Design review of the part built by this model. Coordinates are the model's own, in mm. A direction names the side the tool comes from. Give positions to 0.01 mm unless a question says otherwise; leave off trailing zeros. Write each loop counter-clockwise with the first axis right and the second up, starting at its lowest first coordinate (ties: lowest second). Pieces come first, ordered by that corner, then holes. Notation, with made-up numbers: (16.25, 63) -> (51.25, 63) arc R27 cw to (51.25, 95) -> close; hole circle Ø11 at (13, -32.75). An arc over 180 degrees is marked (long way). Return JSON: item names as keys, results as strings. Group by question number.
from build123d import *

# Parameters (mm, degrees)
SZKIC1_R                    = 9.42
DODANIE_WYCI_GNI_CIE1_DEPTH = 1.34
SZKIC2_R                    = 8.4
DODANIE_WYCI_GNI_CIE2_DEPTH = 3.92
SZKIC3_R                    = 10.19
DODANIE_WYCI_GNI_CIE3_DEPTH = 2.76
SZKIC4_R                    = 8.4
DODANIE_WYCI_GNI_CIE4_DEPTH = 3.92
SZKIC5_R                    = 9.42
DODANIE_WYCI_GNI_CIE5_DEPTH = 1.18
SZKIC6_R                    = 7.5
WYTNIJ_WYCI_GNI_CIE1_DEPTH  = 8.9
WYTNIJ_WYCI_GNI_CIE2_REACH  = 15.12
SZKIC7_R                    = 1.5
CROQUIS1_R                  = 5
CROQUIS1_R_2                = 1.5
SALIENTE_EXTRUIR1_DEPTH     = 5
CROQUIS2_R                  = 0.635
CORTAR_EXTRUIR1_DEPTH       = 11.19
CORTAR_EXTRUIR1_DEPTH_BACK  = 11.19


with BuildPart() as part:
    # Szkic1 → Dodanie-wyciągnięcie1 (new body)
    with BuildSketch(Plane.XY):
        Circle(SZKIC1_R)
    extrude(amount=DODANIE_WYCI_GNI_CIE1_DEPTH)

    # Szkic2 → Dodanie-wyciągnięcie2 (add)
    with BuildSketch(Plane.XY.offset(1.34)):
        Circle(SZKIC2_R)
    extrude(amount=DODANIE_WYCI_GNI_CIE2_DEPTH)

    # Szkic3 → Dodanie-wyciągnięcie3 (add)
    with BuildSketch(Plane.XY.offset(5.26)):
        Circle(SZKIC3_R)
    extrude(amount=DODANIE_WYCI_GNI_CIE3_DEPTH)

    # Szkic4 → Dodanie-wyciągnięcie4 (add)
    with BuildSketch(Plane.XY.offset(8.02)):
        Circle(SZKIC4_R)
    extrude(amount=DODANIE_WYCI_GNI_CIE4_DEPTH)

    # Szkic5 → Dodanie-wyciągnięcie5 (add)
    with BuildSketch(Plane.XY.offset(11.94)):
        Circle(SZKIC5_R)
    extrude(amount=DODANIE_WYCI_GNI_CIE5_DEPTH)

    # Szkic6 → Wytnij-wyciągnięcie1 (cut)
    with BuildSketch(Plane.XY.offset(13.12)):
        Circle(SZKIC6_R)
    extrude(amount=-WYTNIJ_WYCI_GNI_CIE1_DEPTH, mode=Mode.SUBTRACT)

    # Szkic7 → Wytnij-wyciągnięcie2 (cut, up to next)
    with BuildSketch(Plane(origin=(0, 0, 0), x_dir=(-1, 0, 0), z_dir=(0, 0, -1)), mode=Mode.PRIVATE) as wytnij_wyci_gni_cie2_sk1:
        Circle(SZKIC7_R)
    wytnij_wyci_gni_cie2_tool1 = extrude(wytnij_wyci_gni_cie2_sk1.sketch, amount=-WYTNIJ_WYCI_GNI_CIE2_REACH, mode=Mode.PRIVATE) & part.part
    add(wytnij_wyci_gni_cie2_tool1.solids().sort_by_distance((0, 0, 0))[0], mode=Mode.SUBTRACT)

    # Croquis1 → Saliente-Extruir1 (add)
    with BuildSketch(Plane(origin=(0, 0, 0), x_dir=(-1, 0, 0), z_dir=(0, 0, -1))):
        Circle(CROQUIS1_R)
        Circle(CROQUIS1_R_2, mode=Mode.SUBTRACT)
    extrude(amount=SALIENTE_EXTRUIR1_DEPTH)

    # Croquis2 → Cortar-Extruir1 (cut, two sides)
    with BuildSketch(Plane(origin=(0, 0, 0), x_dir=(1, 0, 0), z_dir=(0, 1, 0))) as cortar_extruir1_sk:
        with Locations((0, 2.367182901)):
            Circle(CROQUIS2_R)
    extrude(amount=CORTAR_EXTRUIR1_DEPTH, mode=Mode.SUBTRACT)
    extrude(cortar_extruir1_sk.sketch, amount=-CORTAR_EXTRUIR1_DEPTH_BACK, mode=Mode.SUBTRACT)


solid = part.part
Q1. Take a section at D-D, the plane y = 6.5. Give the boundary of the cut face in (x, z).
Q2. Mouldability with a two-part tool opening along Y and no side actions: class faces 5 (the face through (-8, 4, 1.34)), 6 (the face through (2, 0, 4.22)), 7 (the face through (-2.209, -9.948, 6.621)), 8 (the face through (-7.493, 0.33, 8.732)) as +Y half, -Y half, draft (parallel to the pull), parting line (faces both ways), or undercut.
Q3. Take a section at C-C, the plane x = 0. Count the separate pieces of the cut face and the enclosed holes in it, plus the area to 3 significant figures.
Q4. Tool access review of faces 1 (the face through (-2.042, -9.196, 0.661)), 2 (the face through (-8, 4, 11.94)), 3 (the face through (-0.138, -3.154, -1.747)), 4 (the face through (-2.042, -9.196, 12.522)): name each direction out of +Z, -Z, +X, -X, +Y, -Y from which nothing blocks a thin tool from reaching the whole face with its end or side.
Q5. For L1, parallel to Y at x = 0, z = 7.75; L2, parallel to Y at x = 0, z = 3.15; L3, parallel to Z at x = 1, y = 4, list the stretches that pass through material, from the lowest coordinate up. Write a range as from..to.
Q6. Take a section at B-B, the plane z = -0.75. Give the boundary of the cut face in (x, y).
Q7. Insertion check: pin 1 (10 mm diameter, centred on x = -2.5, z = -2, fed in from +Y); pin 2 (8 mm diameter, centred on x = 6.5, z = -2.5, fed in from +Y); pin 3 (2 mm diameter, centred on y = 0, z = -3, fed in from -X); pin 4 (6 mm diameter, centred on y = 1.5, z = 5.5, fed in from -X). Each pin has a flat end and moves straight along its axis. Give the tip position at first contact, or say it passes through.
Final values:
{
 "1": {"outline": "(-7.85, 5.26) -> (-5.32, 5.26) -> (-5.32, 1.34) -> (-6.82, 1.34) -> (-6.82, 0) -> (6.82, 0) -> (6.82, 1.34) -> (5.32, 1.34) -> (5.32, 5.26) -> (7.85, 5.26) -> (7.85, 8.02) -> (5.32, 8.02) -> (5.32, 11.94) -> (6.82, 11.94) -> (6.82, 13.12) -> (3.74, 13.12) -> (3.74, 4.22) -> (-3.74, 4.22) -> (-3.74, 13.12) -> (-6.82, 13.12) -> (-6.82, 11.94) -> (-5.32, 11.94) -> (-5.32, 8.02) -> (-7.85, 8.02) -> close"},
 "2": {"face 5": "draft", "face 6": "undercut", "face 7": "parting line", "face 8": "undercut"},
 "3": {"separate pieces": "4", "enclosed holes": "0", "area": "115 mm²"},
 "4": {"face 1": "-Z", "face 2": "none", "face 3": "+Y, -Y", "face 4": "+Z"},
 "5": {"L1": "y = -10.19..-7.5, 7.5..10.19", "L2": "y = -8.4..-1.5, 1.5..8.4", "L3": "z = -5..4.22"},
 "6": {"outline": "circle Ø10 at (0, 0); hole circle Ø3 at (0, 0)"},
 "7": {"pin 1": "stops at y = 9.42", "pin 2": "stops at y = 8.79", "pin 3": "stops at x = -5", "pin 4": "stops at x = -10.19"}
}
